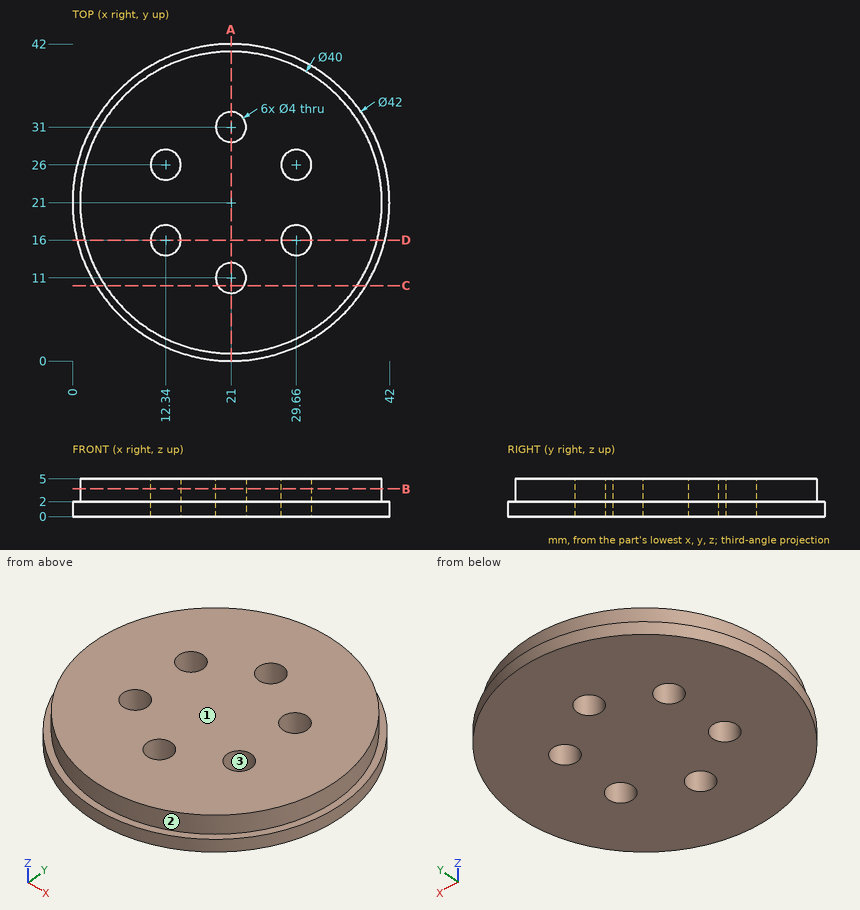
Answer from the drawing. Dimensions are ordinates in mm from the lowest x, y and z of the part. Coordinates: 2 decimals unless noted, no trailing zeros. Write each loop counter-clockwise with the first axis right and the second up, starting at its lowest first coordinate (ties: lowest second). Pieces come first, ordered by that corner, then holes. Notation, with made-up numbers: M -29,-16.5 L 20,-16.5 A14 cw 20,-7.5 Z; hole C 87,56 d1. An arc over 180 degrees is marked long. Put each result on its own line as item: value. Start each with the question number.
1. For a pull along X with two mould halves and no side action, classify the marked faces 1, 2 and 3 as pulls with the +X half, pulls with the -X half, needs draft (parallel to the pull), parting line crosses it, or undercut.
2. A cutting plane is placed at A-A on x = 21. Write down the section's boundary in (y, z), then the cut area to 3 significant figures.
3. A flat-ended cylindrical pin translates along its axis: P1, Ø2, axis at x = 31, z = 4, coming from the +Y side. Find the tip coordinate at first contact, or state that the pin passes through.
4. A cutting plane is placed at B-B on z = 3.7. Write down the section's boundary in (x, y).
5. A cutting plane is placed at C-C on y = 10. Write down the section's boundary in (x, z).
6. Consider line 1 (Y direction, x = 22.5, z = 2.9) (1 decimal); line 2 (Y direction, x = 14, z = 2.65) (1 decimal); line 3 (X direction, y = 16.5, z = 0.3). Determine where each line is inside the solid, lowest interval first. Write a range as from..to.
7. A cutting plane is placed at D-D on y = 16. Write down the section's boundary in (x, z) (1 decimal), then the cut area to 3 significant figures.
Resolved:
1. face 1: needs draft
1. face 2: parting line crosses it
1. face 3: undercut
2. outline: M 0,0 L 9,0 L 9,5 L 1,5 L 1,2 L 0,2 Z; M 13,0 L 29,0 L 29,5 L 13,5 Z; M 33,0 L 42,0 L 42,2 L 41,2 L 41,5 L 33,5 Z
2. area: 164 mm2
3. P1: stops at y = 38.86
4. outline: C 21,21 d40; hole C 12.34,16 d4; hole C 12.34,26 d4; hole C 21,11 d4; hole C 21,31 d4; hole C 29.66,16 d4; hole C 29.66,26 d4
5. outline: M 3.11,0 L 19.27,0 L 19.27,5 L 4.3,5 L 4.3,2 L 3.11,2 Z; M 22.73,0 L 38.89,0 L 38.89,2 L 37.7,2 L 37.7,5 L 22.73,5 Z
6. line 1: y = 1.1..9.7, 12.3..29.7, 32.3..40.9
6. line 2: y = 2.3..14.9, 17.1..24.9, 27.1..39.7
6. line 3: x = 0.49..10.4, 14.28..27.72, 31.6..41.51
7. outline: M 0.6,0 L 10.3,0 L 10.3,5 L 1.6,5 L 1.6,2 L 0.6,2 Z; M 14.3,0 L 27.7,0 L 27.7,5 L 14.3,5 Z; M 31.7,0 L 41.4,0 L 41.4,2 L 40.4,2 L 40.4,5 L 31.7,5 Z
7. area: 158 mm2
